from build123d import *

# Parameters (mm, degrees)
SKETCH1_R           = 22
SKETCH1_R_2         = 2
BOSS_EXTRUDE1_DEPTH = 21.5
SKETCH2_R           = 19
CUT_EXTRUDE1_DEPTH  = 18.5
SKETCH3_R           = 22
SKETCH3_R_2         = 20
CUT_EXTRUDE2_DEPTH  = 1.5


with BuildPart() as part:
    # Sketch1 → Boss-Extrude1 (new body)
    with BuildSketch(Plane.XY):
        Circle(SKETCH1_R)
        Circle(SKETCH1_R_2, mode=Mode.SUBTRACT)
    extrude(amount=BOSS_EXTRUDE1_DEPTH)

    # Sketch2 → Cut-Extrude1 (cut)
    with BuildSketch(Plane.XY.offset(21.5)):
        Circle(SKETCH2_R)
    extrude(amount=-CUT_EXTRUDE1_DEPTH, mode=Mode.SUBTRACT)

    # Sketch3 → Cut-Extrude2 (cut, symmetric)
    with BuildSketch(Plane.XY.offset(10.75)):
        Circle(SKETCH3_R)
        Circle(SKETCH3_R_2, mode=Mode.SUBTRACT)
    extrude(amount=CUT_EXTRUDE2_DEPTH, both=True, mode=Mode.SUBTRACT)


solid = part.part
Check sheet for the modelled part. Datum: model origin and axes. Units: mm. A direction names the side the tool comes from. Round coordinates to 2 decimals unless told otherwise and drop trailing zeros. Order: outer loops, then holes, each group sorted by start corner. A loop starts at its lowest first (then second) coordinate and runs counter-clockwise, first axis right, second up. Notation, with made-up numbers: M 14.5,27.25 L 22.5,27.25 A19 cw 22.5,56.25 Z; hole C 46,39 d2. An arc over 180 degrees is marked long. One line per item, written item: value. Start each with the question number.
1. Section check C-C on z = 15.5. Enter the section's corners in (x, y).
2. Gauge pin test, flat ends, axial feed: P1, Ø10, axis at y = 1.5, z = 18, coming from the +X side; P2, Ø5, axis at y = 12.5, z = 3, coming from the -X side; P3, Ø3, axis at y = 9.5, z = 17.5, coming from the -X side; P4, Ø5, axis at x = 0, y = 0, coming from the +Z side. Record the tip position at first contact, or that the pin passes through.
3. Access from +Z, -Z, +X, -X, +Y, -Y to the whole of each face (thin tool, end or side, straight path). Record for faces 1 (the flat face through (0, -4, 3)), 2 (the cylindrical face through (-4.769, -21.477, 16.81)), 3 (the flat face through (10, -18, 12.25)).
4. Scan lines: line 1 along Y through (x, z) = (0, 2.3); line 2 along Z through (x, y) = (18.5, -9.5); line 3 along Y through (x, z) = (0, 7). Record each from-to range of solid material in increasing order.
5. Section check A-A on x = 0. Enter the section's corners in (y, z).
6. Release check for a two-part mould opening along Z. For faces 4 (the flat face through (-7, 18, 21.5)), 5 (the flat face through (10, -18, 9.25)), 6 (the cylindrical face through (0, -2, 1)) record: released by +Z, released by -Z, zero draft, split by the parting line, or undercut.
7. Section check D-D on y = 14.5. Enter the section's corners in (x, z).
Results found:
1. outline: C 0,0 d44; hole C 0,0 d38
2. P1: x = 22
2. P2: x = -19.6
2. P3: x = -20.49
2. P4: z = 3
3. face 1: +Z
3. face 2: +Z, -Z
3. face 3: none
4. line 1: -22 to -2, 2 to 22
4. line 2: 0 to 9.25, 12.25 to 21.5
4. line 3: -22 to -19, 19 to 22
5. outline: M -22,0 L -2,0 L -2,3 L -19,3 L -19,21.5 L -22,21.5 L -22,12.25 L -20,12.25 L -20,9.25 L -22,9.25 Z; M 2,0 L 22,0 L 22,9.25 L 20,9.25 L 20,12.25 L 22,12.25 L 22,21.5 L 19,21.5 L 19,3 L 2,3 Z
6. face 4: released by +Z
6. face 5: undercut
6. face 6: zero draft
7. outline: M -16.55,0 L 16.55,0 L 16.55,9.25 L 13.77,9.25 L 13.77,12.25 L 16.55,12.25 L 16.55,21.5 L 12.28,21.5 L 12.28,3 L -12.28,3 L -12.28,21.5 L -16.55,21.5 L -16.55,12.25 L -13.77,12.25 L -13.77,9.25 L -16.55,9.25 Z
